Check sheet for the drawn part. Datum: minimum x, y, z corner. Units: mm. Round coordinates to 2 decimals unless told otherwise and drop trailing zeros. Write each loop counter-clockwise with the first axis right and the second up, starting at its lowest first coordinate (ties: lowest second). Pieces come first, ordered by that corner, then holes. Notation, with made-up numbers: (1, 67) - (35, 67) arc R8 ccw to (35, 74) - close; hole circle Ø4 at (57.5, 71.25). An arc over 180 degrees is marked (long way). Answer as a JSON object with one key per item and string values. Group by question number.
1) Go/stop test with flat-tipped pins: pin 1 Ø12 at (x, y) = (4, 9.5) entering from +Z; pin 2 Ø4 at (y, z) = (21.5, 173.5) entering from -X; pin 3 Ø1.5 at (x, y) = (16, 4.5) entering from +Z; pin 4 Ø1 at (x, y) = (17.5, 7) entering from -Z. Record where each tip stops, or that it passes through.
2) Section check B-B (x = 19). Enter the section's corners in (y, z), then the cut area to 3 significant figures.
3) Section check A-A (y = 12.7). Enter the section's corners in (x, z) (3 decimals).
4) Section check C-C (z = 106). Enter the section's corners in (x, y) (3 decimals).
5) Thickness scan on line 1 (Z direction, x = 31, y = 12.7); line 2 (Y direction, x = 27.75, z = 393.7); line 3 (X direction, y = 8.5, z = 238) (3 decimals). Record the ranges inside material, lowest first.
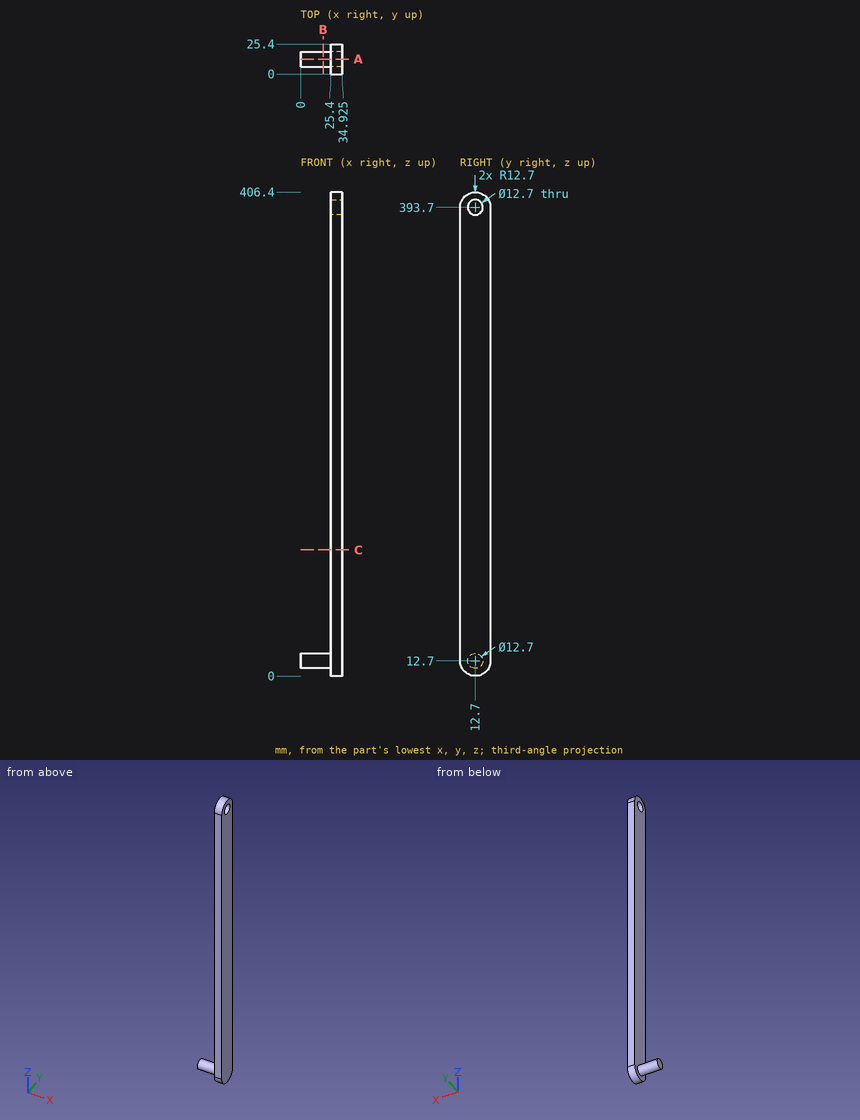
Returned:
{
 "1": {"pin 1": "z = 19.05", "pin 2": "x = 25.4", "pin 3": "through", "pin 4": "z = 9.06"},
 "2": {"outline": "circle Ø12.7 at (12.7, 12.7)", "area": "127 mm2"},
 "3": {"outline": "(0, 6.35) - (25.4, 6.35) - (25.4, 0) - (34.925, 0) - (34.925, 387.35) - (25.4, 387.35) - (25.4, 19.05) - (0, 19.05) - close; (25.4, 400.05) - (34.925, 400.05) - (34.925, 406.4) - (25.4, 406.4) - close"},
 "4": {"outline": "(25.4, 0) - (34.925, 0) - (34.925, 25.4) - (25.4, 25.4) - close"},
 "5": {"line 1": "0 to 387.35, 400.05 to 406.4", "line 2": "0 to 6.35, 19.05 to 25.4", "line 3": "25.4 to 34.925"}
}
